Geometry check sheet. Reference: drawing and pictorial views, mm from the part's lowest x, y, z. A direction names the side the tool comes from. Coordinates: 2 decimals unless noted, no trailing zeros. Write each loop counter-clockwise with the first axis right and the second up, starting at its lowest first coordinate (ties: lowest second). Pieces come first, ordered by that corner, then holes. Notation, with made-up numbers: (38, -9) - (85, -9) arc R11 ccw to (85, 7) - close; hole circle Ø6 at (-13, 68). An arc over 180 degrees is marked (long way). Use one line per item in the form item = value. Start each with the question number.
(1) Mould release check, pull along X, two halves, no side actions. Record for the marked faces 1, 2, 3 and 4: released by +X, released by -X, zero draft, split by the parting line, or undercut.
(2) Gauge pin test, flat end, axial feed: pin 1 Ø4 at (x, z) = (261.5, 648) entering from -Y. Record the tip position at first contact, or that the pin passes through.
(3) Sectioned sample at C-C (z = 877). Record the cut outline in (x, y), and give its area (3 significant figures).
(4) Sectioned sample at A-A (y = 242). Record the cut outline in (x, z).
(5) Sectioned sample at D-D (x = 91.5). Record the cut outline in (y, z), and give its area (3 significant figures).
(6) Tool access check on the marked faces 5 and 6. Record the directions out of +Z, -Z, +X, -X, +Y, -Y that give a thin tool (end or side, any length) a straight path to the whole face; none if there is none.
(7) Sectioned sample at B-B (x = 763.5). Record the cut outline in (y, z).
(8) Material ranges on line 1 (X direction, y = 268, z = 540.5); line 2 (Z direction, x = 188, y = 323.5); line 3 (Z direction, x = 1033.5, y = 61.5), recorded low to high. Write a range as [from, to].
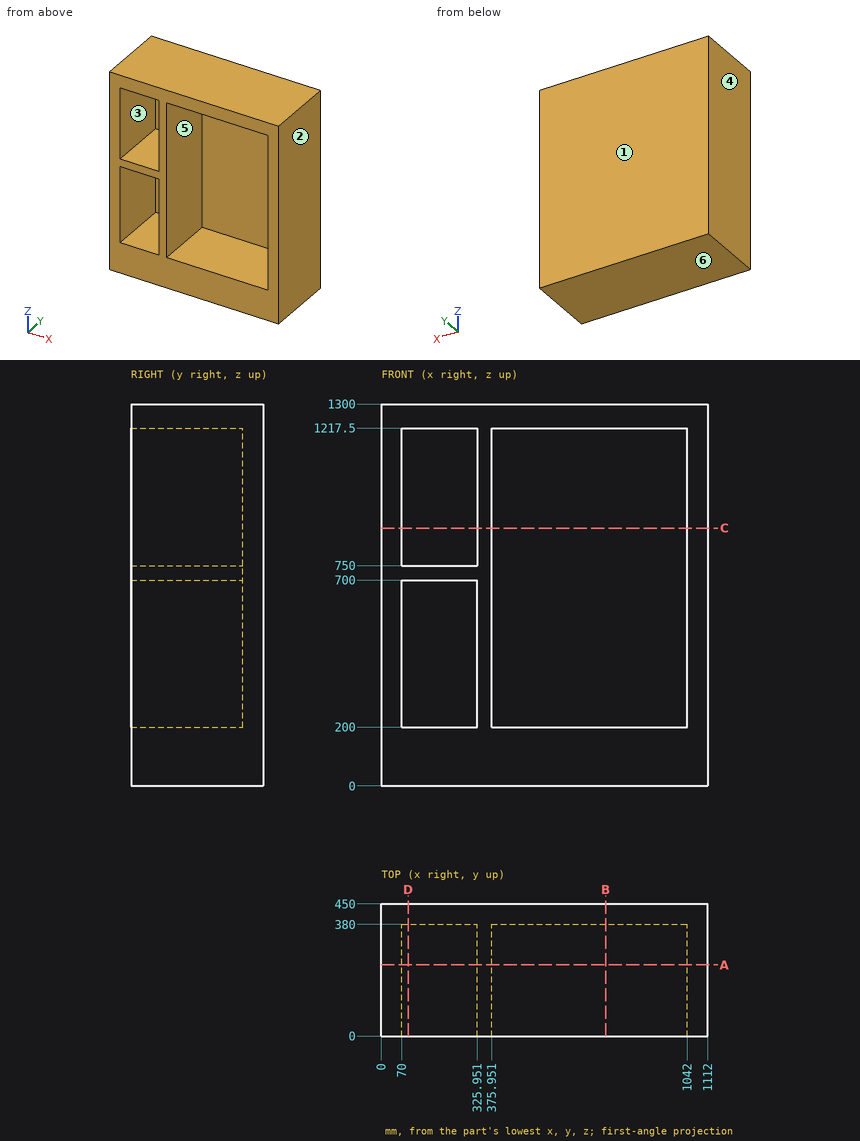
Answers below:
q1.face_1 = zero draft
q1.face_2 = released by +X
q1.face_3 = undercut
q1.face_4 = released by -X
q2.pin_1 = 380
q3.outline = (0, 0) - (70, 0) - (70, 380) - (325.95, 380) - (325.95, 0) - (375.95, 0) - (375.95, 380) - (1042, 380) - (1042, 0) - (1112, 0) - (1112, 450) - (0, 450) - close
q3.area = 150,000 mm2
q4.outline = (0, 0) - (1112, 0) - (1112, 1300) - (0, 1300) - close; hole (70, 200) - (325.95, 200) - (325.95, 700) - (70, 700) - close; hole (70, 750) - (325.95, 750) - (325.95, 1217.5) - (70, 1217.5) - close; hole (375.95, 200) - (1042, 200) - (1042, 1217.5) - (375.95, 1217.5) - close
q5.outline = (0, 0) - (450, 0) - (450, 1300) - (0, 1300) - (0, 1217.5) - (380, 1217.5) - (380, 750) - (0, 750) - (0, 700) - (380, 700) - (380, 200) - (0, 200) - close
q5.area = 217,000 mm2
q6.face_5 = -Y
q6.face_6 = -Z, +X, -X, +Y, -Y
q7.outline = (0, 0) - (450, 0) - (450, 1300) - (0, 1300) - (0, 1217.5) - (380, 1217.5) - (380, 200) - (0, 200) - close
q8.line_1 = [0, 70], [325.95, 375.95], [1042, 1112]
q8.line_2 = [0, 200], [700, 750], [1217.5, 1300]
q8.line_3 = [0, 200], [1217.5, 1300]
